from build123d import *

# Parameters (mm, degrees)
CUT_EXTRUDE1_DEPTH  = 33
BOSS_EXTRUDE2_START = -6.898371775
SKETCH3_W           = 18
SKETCH3_H           = 0.818990312
BOSS_EXTRUDE2_DEPTH = 10.555064026
SKETCH4_W           = 8
SKETCH4_H           = 3
BOSS_EXTRUDE3_DEPTH = 21
SKETCH6_W           = 8
SKETCH6_H           = 5.661156415
BOSS_EXTRUDE4_DEPTH = 15
SKETCH7_W           = 17.96730976
SKETCH7_H           = 0.5
BOSS_EXTRUDE7_DEPTH = 11


with BuildPart() as part:
    # Sketch1 → Revolve1 (revolve)
    with BuildSketch(Plane.XY):
        with BuildLine():
            Line((-26.25, 0), (-28.5, 0))
            ThreePointArc((-28.5, 0), (-20.152543264, -20.152543264), (0, -28.5))
            Line((0, -28.5), (0, -25))
            ThreePointArc((0, -25), (-16.007810594, -19.20286437), (-24.591665255, -4.5))
            Line((-24.591665255, -4.5), (-26.25, -4.5))
            Line((-26.25, -4.5), (-26.25, 0))
        make_face()
    revolve(axis=Axis((0, 0, 0), (0, -1, 0)))

    # Sketch2 → Cut-Extrude1 (cut)
    with BuildSketch(Plane(origin=(0, 0, 0), x_dir=(1, 0, 0), z_dir=(0, 1, 0))):
        Polygon((-5, -9.5), (-5, -5.5), (5, -5.5), (5, -9.5), (11, -9.5), (11, -11), (-11, -11), (-11, -9.5), align=None)
    extrude(amount=-CUT_EXTRUDE1_DEPTH, mode=Mode.SUBTRACT)

    # Sketch3 → Boss-Extrude2 (add)
    with BuildSketch(Plane(origin=(0, -4.5, 0), x_dir=(1, 0, 0), z_dir=(0, 1, 0)).offset(BOSS_EXTRUDE2_START)):
        with Locations((0, -12.409495156)):
            Rectangle(SKETCH3_W, SKETCH3_H)
    extrude(amount=-BOSS_EXTRUDE2_DEPTH)

    # Sketch4 → Boss-Extrude3 (add)
    with BuildSketch(Plane(origin=(0, -4.5, 0), x_dir=(1, 0, 0), z_dir=(0, 1, 0))):
        with Locations((0, 9.5)):
            Rectangle(SKETCH4_W, SKETCH4_H)
    extrude(amount=-BOSS_EXTRUDE3_DEPTH)

    # Sketch6 → Boss-Extrude4 (add)
    with BuildSketch(Plane(origin=(0, 0, -11), x_dir=(-1, 0, 0), z_dir=(0, 0, -1))):
        with Locations((0, -7.330578208)):
            Rectangle(SKETCH6_W, SKETCH6_H)
    extrude(amount=BOSS_EXTRUDE4_DEPTH)

    # Sketch7 → Boss-Extrude7 (add)
    with BuildSketch(Plane.XY.offset(12.818990312)):
        with Locations((0.01634512, -11.648371775)):
            Rectangle(SKETCH7_W, SKETCH7_H)
    extrude(amount=BOSS_EXTRUDE7_DEPTH)


solid = part.part
Check sheet for the modelled part. Datum: model origin and axes. Units: mm. A direction names the side the tool comes from. Round coordinates to 2 decimals unless told otherwise and drop trailing zeros. Write each loop counter-clockwise with the first axis right and the second up, starting at its lowest first coordinate (ties: lowest second). Pieces come first, ordered by that corner, then holes. Notation, with made-up numbers: (46.25, 15.25) - (54.25, 15.25) arc R16 ccw to (54.25, 44.25) - close; hole circle Ø4 at (85.25, 4). An arc over 180 degrees is marked (long way). Return JSON: item names as keys, results as strings.
Q1. Depth check by flat-ended pin: P1, Ø1.2, axis at y = -24.5, z = 7.5, coming from the +X side; P2, Ø3, axis at y = -5.5, z = 19.5, coming from the +X side; P3, Ø8, axis at x = -9, y = -17, coming from the -Z side. Enter the tip coordinate at first touch or a pass-through.
Returned:
{"P1": "stops at x = 13.64", "P2": "stops at x = 21.45", "P3": "stops at z = -24.09"}
Q2. Access from +Z, -Z, +X, -X, +Y, -Y to the whole of each face (thin tool, end or side, straight path). Record for faces 1 (the flat face through (0, -10.161, -17)), 2 (the flat face through (4, -10, -14)), 3 (the flat face through (-11, -22, 10)).
Returned:
{"face 1": "none", "face 2": "+Y", "face 3": "+Y, -Y"}
Q3. Cross-section at B-B (z = 6.5). Record the boundary of the cut face in (x, y).
Returned:
{"outline": "(-27.75, 0) arc R27.75 ccw to (-5, -27.29) - (-5, -23.62) arc R24.14 cw to (-23.72, -4.5) - (-25.43, -4.5) - (-25.43, 0) - close; (5, -27.29) arc R27.75 ccw to (27.75, 0) - (25.43, 0) - (25.43, -4.5) - (23.72, -4.5) arc R24.14 cw to (5, -23.62) - close"}
Q4. Draft check along Y on faces 4 (the flat face through (13, 0, 23)), 5 (the flat face through (0, -16, -11)), 6 (the flat face through (0, -11.898, 17)), 7 (the flat face through (-8, -23, 9.5)). Enter one of: released by +Y, released by -Y, zero draft, split by the parting line, or undercut.
Returned:
{"face 4": "released by +Y", "face 5": "undercut", "face 6": "undercut", "face 7": "zero draft"}
Q5. Cross-section at C-C (x = -6.5). Record the boundary of the cut face in (y, z).
Returned:
{"outline": "(-26.07, 9.5) arc R27.75 ccw to (0, -27.75) - (0, -25.43) - (-4.5, -25.43) - (-4.5, -23.72) arc R24.14 cw to (-22.19, 9.5) - close; (-25.48, 11) - (-21.49, 11) arc R24.14 cw to (-20.95, 12) - (-11.4, 12) - (-11.4, 21.28) arc R24.14 cw to (-4.5, 23.72) - (-4.5, 25.43) - (0, 25.43) - (0, 27.75) arc R27.75 ccw to start; hole (-20.46, 12.82) - (-11.9, 12.82) - (-11.9, 21) arc R24.14 ccw to start"}
Q6. Scan lines: L1, parallel to X at y = -2.5, z = 3.5; L2, parallel to Y at x = -3, z = -20; L3, parallel to X at y = -3.4, z = 0. Record each from-to range of solid material in increasing order. Write a range as from..to.
Returned:
{"L1": "x = -28.17..-26.02, 26.02..28.17", "L2": "y = -20.08..-14.7, -10.16..-4.5", "L3": "x = -28.3..-26.25, 26.25..28.3"}
Q7. Cross-section at D-D (z = 0). Record the boundary of the cut face in (x, y), then the cut area to 3 significant figures.
Returned:
{"outline": "(-28.5, 0) arc R28.5 ccw to (28.5, 0) - (26.25, 0) - (26.25, -4.5) - (24.59, -4.5) arc R25 cw to (-24.59, -4.5) - (-26.25, -4.5) - (-26.25, 0) - close", "area": "282 mm²"}
Q8. Cross-section at A-A (x = 0). Record the boundary of the cut face in (y, z).
Returned:
{"outline": "(-27.96, 5.5) arc R28.5 ccw to (0, -28.5) - (0, -26.25) - (-4.5, -26.25) - (-4.5, -8) - (-23.69, -8) arc R25 cw to (-24.39, 5.5) - close; (-26.29, 11) - (-22.45, 11) arc R25 cw to (-21.93, 12) - (-11.4, 12) - (-11.4, 22.25) arc R25 cw to (-4.5, 24.59) - (-4.5, 26.25) - (0, 26.25) - (0, 28.5) arc R28.5 ccw to start; hole (-22.45, -11) arc R25 ccw to (-10.16, -22.84) - (-10.16, -11) - close; hole (-21.46, 12.82) - (-11.9, 12.82) - (-11.9, 21.99) arc R25 ccw to start"}
